```python
from build123d import *

# Parameters (mm, degrees)
SKETCH_1_R          = 3.35
EXTRUDE_1_DEPTH     = 10.5
EXTRUDE_1_DRAFT     = -6.5
SKETCH_2_R          = 3
CUT_EXTRUDE_1_DEPTH = 9
FILLET_1_R          = 1
FILLET_2_R          = 0.2


with BuildPart() as part:
    # Эскиз1 → Бобышка-Вытянуть1 (with draft: the straight prism first)
    with BuildSketch(Plane(origin=(0, 0, 0), x_dir=(1, 0, 0), z_dir=(0, 1, 0))):
        Circle(SKETCH_1_R)
    extrude(amount=EXTRUDE_1_DEPTH)
    # Бобышка-Вытянуть1: the draft: its side faces are tilted about the plane it starts from
    extrude_1_sides = [part.faces().sort_by_distance(p)[0] for p in [
        (-3.35, 5.25, 0),
    ]]
    draft(extrude_1_sides, Plane(origin=(0, 0, 0), x_dir=(1, 0, 0), z_dir=(0, 1, 0)), EXTRUDE_1_DRAFT)

    # Эскиз2 → Вырез-Вытянуть1 (cut)
    with BuildSketch(Plane.XZ):
        with Locations(Location((0, 0, 0), (0, 0, 270))):
            Circle(SKETCH_2_R)
    extrude(amount=-CUT_EXTRUDE_1_DEPTH, mode=Mode.SUBTRACT)

    # Скругление1
    fillet_1_edges = [part.edges().sort_by_distance(p)[0] for p in [
        (-4.546323887, 10.5, 0),
    ]]
    fillet(fillet_1_edges, radius=FILLET_1_R)

    # Скругление2
    fillet_2_edges = [part.edges().sort_by_distance(p)[0] for p in [
        (-3.35, 0, 0),
    ]]
    fillet(fillet_2_edges, radius=FILLET_2_R)


solid = part.part
```
Verification items for the finished model (mm, model axes). Coordinates: 2 decimals unless noted, no trailing zeros. Write each loop counter-clockwise with the first axis right and the second up, starting at its lowest first coordinate (ties: lowest second). Pieces come first, ordered by that corner, then holes. Notation, with made-up numbers: (62.25, -28.75) - (99.25, -28.75) arc R9 ccw to (99.25, -19.75) - close; hole circle Ø3 at (35.25, -19.5). An arc over 180 degrees is marked (long way). One line per question, with ' | ' between items. Start each with the question number.
1. Gauge pin test, flat ends, axial feed: P1, Ø3.5, axis at x = 0, z = 0, coming from the -Y side; P2, Ø1, axis at y = 7.5, z = -3, coming from the +X side; P3, Ø1.5, axis at x = 2, y = 8, coming from the +Z side. Record the tip position at first contact, or that the pin passes through.
2. Draft check along X on faces 1 (the flat face through (0, 10.5, 0)), 2 (the flat face through (0, 9, 0)), 3 (the conical face through (-0.843, 4.718, 3.795)). Enter one of: released by +X, released by -X, zero draft, split by the parting line, or undercut.
3. Section check B-B (z = 0). Enter the section's corners in (x, y), plus the area to 3 significant figures.
4. Section check D-D (y = 9.75). Enter the section's corners in (x, z).
5. Section check C-C (y = 1.5). Enter the section's corners in (x, z), plus the area to 3 significant figures.
6. Section check A-A (x = 0). Enter the section's corners in (y, z).
7. Material ranges on line 1 along Y through (x, z) = (1.5, -1.5); line 2 along X through (y, z) = (2.5, 0); line 3 along Z through (x, y) = (0.75, 1.25), recorded low to high.
Computed values:
1) P1: y = 9 | P2: x = 3.39 | P3: z = 4.09
2) face 1: zero draft | face 2: undercut | face 3: split by the parting line
3) outline: (-4.42, 9.39) - (-3.37, 0.18) arc R0.2 ccw to (-3.17, 0) - (-3, 0) - (-3, 9) - (3, 9) - (3, 0) - (3.17, 0) arc R0.2 ccw to (3.37, 0.18) - (4.42, 9.39) arc R1 ccw to (3.43, 10.5) - (-3.43, 10.5) arc R1 ccw to start | area: 28.3 mm²
4) outline: circle Ø8.79 at (0, 0)
5) outline: circle Ø7.04 at (0, 0); hole circle Ø6 at (0, 0) | area: 10.7 mm²
6) outline: (0, -3.17) arc R0.2 ccw to (0.18, -3.37) - (9.39, -4.42) arc R1 ccw to (10.5, -3.43) - (10.5, 3.43) arc R1 ccw to (9.39, 4.42) - (0.18, 3.37) arc R0.2 ccw to (0, 3.17) - (0, 3) - (9, 3) - (9, -3) - (0, -3) - close
7) line 1: 9 to 10.5 | line 2: -3.63 to -3, 3 to 3.63 | line 3: -3.41 to -2.9, 2.9 to 3.41
